Autodesk Inventor part; units mm, degrees
ref_plane "YZ Plane" through (0, 0, 0) normal (1, 0, 0) x (0, 1, 0)
ref_plane "XZ Plane" through (0, 0, 0) normal (0, 1, 0) x (-1, 0, 0)
ref_plane "XY Plane" through (0, 0, 0) normal (0, 0, 1) x (1, 0, 0)
sketch "Sketch1" plane through (0, 0, 0) normal (0, 1, 0) x (-1, 0, 0)
  circle A0 centre (0, 0) radius 65
  circle A1 centre (0, 0) radius 55
  dimension "d0" = 130
  dimension "d1" = 110
extrude "Extrusion1" add sketch "Sketch1" along normal blind 3
sketch "Sketch2" plane through (0, 3, 0) normal (0, 1, 0) x (1, 0, 0)
  line L0 (-65, -1.5) -> (-56, -1.5)
  line L1 (-56, -1.5) -> (-56, 1.5)
  line L2 (-56, 1.5) -> (-65, 1.5)
  line L3 (-65, 1.5) -> (-65, -1.5)
  point P0 (0, 0)
  dimension "d4" = 3
  dimension "d5" = 9
  dimension "d6" = 1.5
  dimension "d7" = 65
extrude "Extrusion2" cut sketch "Sketch2" against normal blind 10
pattern_circular "Circular Pattern1" count 6 over 360 about axis through (0, -10, 0) along (0, 1, 0) of "Extrusion2"
properties part number "os"
The model under review builds one solid part; all positions refer to its coordinate system, in mm. A direction names the side the tool comes from. Coordinates: 2 decimals unless noted, no trailing zeros. Write each loop counter-clockwise with the first axis right and the second up, starting at its lowest first coordinate (ties: lowest second). Pieces come first, ordered by that corner, then holes. Notation, with made-up numbers: M -29,-29 L -22,-29 A29 cw -22,0 Z; hole C 11.25,79.25 d5. An arc over 180 degrees is marked long. Put each result on its own line as item: value.
1) Wall thickness on probe 1 along Z at (x, y) = (-1.5, 0.35); probe 2 along Z at (x, y) = (-28.5, 2.8); probe 3 along Z at (x, y) = (29.5, 2.75): over which ranges is each line inside the solid? List them lowest first. Write a range as [from, to].
Computed:
probe 1: z = [-64.98, -54.98], [54.98, 64.98]
probe 2: z = [-58.42, -52.36], [-48.21, -47.04], [47.04, 48.21], [52.36, 58.42]
probe 3: z = [-57.92, -54.1], [-48.1, -46.42], [46.42, 48.1], [54.1, 57.92]
2) Add section C-C on y = 1.3. Give the boundary of the cut face in (x, z), then the cut area to 3 significant figures.
Computed:
outline: M -64.98,-1.5 A65 ccw -33.79,-55.53 L -29.3,-47.75 L -26.7,-49.25 L -31.19,-57.03 A65 ccw 31.19,-57.03 L 26.7,-49.25 L 29.3,-47.75 L 33.79,-55.53 A65 ccw 64.98,-1.5 L 56,-1.5 L 56,1.5 L 64.98,1.5 A65 ccw 33.79,55.53 L 29.3,47.75 L 26.7,49.25 L 31.19,57.03 A65 ccw -31.19,57.03 L -26.7,49.25 L -29.3,47.75 L -33.79,55.53 A65 ccw -64.98,1.5 L -56,1.5 L -56,-1.5 Z; hole C 0,0 d110
area: 3,610 mm2
3) For faces 1 (the flat face through (-60, 2, -1.5)), 2 (the flat face through (60, 2, 1.5)), 3 (the flat face through (-31.576, 1.521, -51.691)), list the 3-axis set-ups (+Z, -Z, +X, -X, +Y, -Y) from which the entire face can be reached by the end or side of a thin tool; tool diameter is ignored.
Computed:
face 1: -X, +Y, -Y
face 2: +X, +Y, -Y
face 3: +Y, -Y
4) Add section A-A on z = 0. Give the boundary of the cut face in (x, y), then the cut area to 3 significant figures.
Computed:
outline: M -56,0 L -55,0 L -55,3 L -56,3 Z; M 55,0 L 56,0 L 56,3 L 55,3 Z
area: 6.00 mm2
5) Add section B-B on x = 0. Give the boundary of the cut face in (y, z).
Computed:
outline: M 0,-65 L 3,-65 L 3,-55 L 0,-55 Z; M 0,55 L 3,55 L 3,65 L 0,65 Z
6) Clearance check with flat-ended pins moving along their axes: pin 1 Ø1.5 at (y, z) = (0.5, 16) entering from +X; pin 2 Ø0.9 at (x, y) = (58.5, 2) entering from +Z. State where each tip first meets the part, or that it passes through.
Computed:
pin 1: stops at x = 63.19
pin 2: stops at z = 29.24
7) Draft analysis for pull direction X (two halves, no side actions). For faces 4 (the flat face through (-28.978, 1.521, 53.191)), 5 (the cylindrical face through (56, 1, -33)), 6 (the cylindrical face through (0, 1, 65)), state which applies: released by +X, released by -X, zero draft, split by the parting line, or undercut.
Computed:
face 4: undercut
face 5: released by +X
face 6: split by the parting line
